The model under review builds one solid part; all positions refer to its coordinate system, in mm. A direction names the side the tool comes from. Round coordinates to 2 decimals unless told otherwise and drop trailing zeros. Write each loop counter-clockwise with the first axis right and the second up, starting at its lowest first coordinate (ties: lowest second). Pieces come first, ordered by that corner, then holes. Notation, with made-up numbers: (61, 15) -> (85, 15) arc R16 cw to (85, 33) -> close; hole circle Ø6 at (28, 41). An arc over 180 degrees is marked (long way). Return JSON: item names as keys, results as strings. Group by question number.
1. Mouldability with a two-part tool opening along X and no side actions: class faces 1 (the flat face through (2, 5.51, 2)), 2 (the cylindrical face through (0.163, 1.016, -17.448)), 3 (the cylindrical face through (-0.03, 1.02, -21.84)) as pulls with the +X half, pulls with the -X half, needs draft (parallel to the pull), parting line crosses it, or undercut.
2. For line 1 along Z through (x, y) = (0, 2.25) (3 decimals); line 2 along X through (y, z) = (3.6, 0) (3 decimals); line 3 along Y through (x, z) = (-1.75, 1.75), list the stretches that pass through material, from the lowest coordinate up. Write a range as from..to.
3. Clearance check with flat-ended pins moving along their axes: P1, Ø4, axis at x = 0, z = 0, coming from the +Y side; P2, Ø2, axis at x = 0, z = -13.28, coming from the +Y side; P3, Ø2, axis at y = 1.5, z = -7.5, coming from the -X side. State where each tip first meets the part, or that it passes through.
4. Take a section at C-C, the plane y = 3.2. Write out the cut boundary in (x, z) (3 decimals).
5. Tool access review of faces 4 (the cylindrical face through (0.098, 1.016, -21.374)), 5 (the cylindrical face through (0.78, 1.02, 3.52)), 6 (the flat face through (1, 2.7, -1)): name each direction out of +Z, -Z, +X, -X, +Y, -Y from which nothing blocks a thin tool from reaching the whole face with its end or side.
6. Take a section at D-D, the plane y = 1.45. Write out the cut boundary in (x, z) (3 decimals).
7. Take a section at B-B, the plane z = -13.28. Write out the cut boundary in (x, y), then the cut area to 3 significant figures.
Autodesk Inventor part; units mm, degrees
ref_plane "YZ Plane" through (0, 0, 0) normal (1, 0, 0) x (0, 1, 0)
ref_plane "XZ Plane" through (0, 0, 0) normal (0, 1, 0) x (-1, 0, 0)
ref_plane "XY Plane" through (0, 0, 0) normal (0, 0, 1) x (1, 0, 0)
sketch "Sketch1" plane through (0, 0, 0) normal (0, 1, 0) x (-1, 0, 0)
  circle A0 centre (0, 0) radius 4.235
  circle A1 centre (0, 0) radius 2.375
  circle A2 centre (0, 0) radius 1.11
  circle A3 centre (0, 0) radius 3.6056
  arc A4 (-1.21, -20.63) -> (1.21, -20.63) centre (0, -20.63) ccw
  line L0 (-3.38, -2.5516) -> (-1.21, -20.63)
  line L1 (3.38, -2.5516) -> (1.21, -20.63)
  circle A5 centre (0, -20.63) radius 0.75
  circle A6 centre (0, -18.18) radius 0.75
  circle A7 centre (0, -10.83) radius 0.75
  circle A8 centre (0, -13.28) radius 0.75
  circle A9 centre (0, -15.73) radius 0.75
  point P0 (0, -2.5516)
  dimension "d2" = 2.22
  dimension "d3" = 0.6294
  dimension "d14" = 1.5
  dimension "d15" = 0.46
  dimension "d16" = 1.5
  dimension "d17" = 0.95
  dimension "d18" = 1.5
  dimension "d19" = 1.5
  dimension "d20" = 1.5
  dimension "d21" = 0.95
  dimension "d22" = 0.95
  dimension "d23" = 0.95
  dimension "d26" = 4.75
extrude "Extrusion1" add sketch "Sketch1" along normal blind 2.07 contours A0
sketch "Sketch2" plane through (0, 2.07, 0) normal (0, 1, 0) x (1, 0, 0)
  circle A0 centre (0, 0) radius 3.6056
  circle A1 centre (0, 0) radius 2.375
  circle A2 centre (0, 0) radius 3.6056
  circle A3 centre (0, 0) radius 4.235
  circle A4 centre (0, 0) radius 1.11
extrude "Extrusion2" add sketch "Sketch2" along normal blind 0.63 contours A0 | A1 | A3
sketch "Sketch3" plane through (0, 2.7, 0) normal (0, 1, 0) x (1, 0, 0)
  circle A0 centre (0, 0) radius 2.375
  circle A1 centre (0, 0) radius 3.6056
  circle A2 centre (0, 0) radius 4.235
  circle A3 centre (0, 0) radius 1.11
extrude "Extrusion3" add sketch "Sketch3" along normal blind 2.81 contours A1 | A2
extrude "Extrusion4" add sketch "Sketch1" along normal blind 2.06 contours A0 L1 A4 L0
properties part number "hornminiservo"
Output:
{
 "1": {"face 1": "needs draft", "face 2": "undercut", "face 3": "parting line crosses it"},
 "2": {"line 1": "z = -4.235..-1.11, 1.11..4.235", "line 2": "x = -4.235..-2.375, 2.375..4.235", "line 3": "y = 2.07..5.51"},
 "3": {"P1": "stops at y = 2.7", "P2": "stops at y = 2.06", "P3": "stops at x = -2.91"},
 "4": {"outline": "circle Ø8.47 at (0, 0); hole circle Ø4.75 at (0, 0)"},
 "5": {"face 4": "+Y, -Y", "face 5": "-Y", "face 6": "+Y"},
 "6": {"outline": "(-3.38, -2.552) -> (-1.21, -20.63) arc R1.21 ccw to (1.21, -20.63) -> (3.38, -2.552) arc R4.235 ccw (long way) to start; hole circle Ø7.211 at (0, 0); hole circle Ø1.5 at (0, -20.63); hole circle Ø1.5 at (0, -18.18); hole circle Ø1.5 at (0, -15.73); hole circle Ø1.5 at (0, -13.28); hole circle Ø1.5 at (0, -10.83)"},
 "7": {"outline": "(-2.09, 0) -> (-0.75, 0) -> (-0.75, 2.06) -> (-2.09, 2.06) -> close; (0.75, 0) -> (2.09, 0) -> (2.09, 2.06) -> (0.75, 2.06) -> close", "area": "5.53 mm^2"}
}
